from build123d import *

# Parameters (mm, degrees)
CYLINDER001_R     = 8
CYLINDER001_DEPTH = 20
CYLINDER_R        = 11.2
CYLINDER_DEPTH    = 10


with BuildPart() as cylinder001:
    # Cylinder001 → Cylinder001 (new body)
    with BuildSketch(Plane.XY):
        Circle(CYLINDER001_R)
    extrude(amount=CYLINDER001_DEPTH)


with BuildPart() as cylinder:
    # Cylinder → Cylinder (new body)
    with BuildSketch(Plane.XY):
        Circle(CYLINDER_R)
    extrude(amount=CYLINDER_DEPTH)


with BuildPart() as cut001:
    # Cone → Cone (revolve)
    with BuildSketch(Plane.XZ):
        Polygon((0, 0), (20, 0), (12, 20), (0, 20), align=None)
    revolve(axis=Axis((0, 0, 0), (0, 0, 1)))

    # Cut: cut Cylinder
    add(cylinder.part, mode=Mode.SUBTRACT)

    # Cut001: cut Cylinder001
    add(cylinder001.part, mode=Mode.SUBTRACT)


solid = cut001.part
Source: CAD feature listing. Evaluate the final solid. Frame: model axes, mm. A direction names the side the tool comes from. Coordinates: 2 decimals unless noted, no trailing zeros. Loops run counter-clockwise (first coordinate to the right, second up) from the corner with the lowest first, then second, coordinate; pieces in that order, holes last. Notation, with made-up numbers: (60.25, 1.5) - (85.25, 1.5) arc R32 cw to (85.25, 29.5) - close; hole circle Ø5 at (-32, 43). An arc over 180 degrees is marked (long way). One line per item, written item: value. Start each with the question number.
1. Section A-A (y = 0). Return the cut outline in (x, z).
2. Set-up query: faces 4 (the cylindrical face through (-1.73, -7.81, 14.93)), 5 (the cylindrical face through (-11.19, 0.49, 4.93)). Return all of +Z, -Z, +X, -X, +Y, -Y with unobstructed straight access to the full face (end or side cutting, diameter ignored); none if empty.
3. Contact query for flat-ended pins moving along their axis: P1, Ø6, axis at y = -9.5, z = 16, coming from the +X side; P2, Ø6, axis at x = 10, y = -14, coming from the +Z side; P3, Ø6, axis at x = 1, z = 4, coming from the -Y side; P4, Ø13.5, axis at x = 0, y = 0, coming from the -Z side. Output: stop coordinate, or through.
4. Mould query, pull axis X, two halves, no side actions, for faces 1 (the flat face through (-8, 3, 10)), 2 (the conical face through (-3.07, -13.83, 14.58)), 3 (the flat face through (2, -8, 20)). Classes: pulls with the +X half, pulls with the -X half, needs draft (parallel to the pull), parting line crosses it, or undercut.
5. Section C-C (z = 7.5). Return the cut outline in (x, y), and give its area (3 significant figures).
6. Ray query, L1, parallel to Z at x = -7, y = 8; L2, parallel to Y at x = -9.5, z = 2.75; L3, parallel to X at y = 9, z = 12.5. Return the intervals inside material, ascending.
Verdict:
1. outline: (-20, 0) - (-11.2, 0) - (-11.2, 10) - (-8, 10) - (-8, 20) - (-12, 20) - close; (8, 10) - (11.2, 10) - (11.2, 0) - (20, 0) - (12, 20) - (8, 20) - close
2. face 4: +Z, -Z
2. face 5: -Z
3. P1: stops at x = 12.44
3. P2: stops at z = 14.49
3. P3: stops at y = -19.58
3. P4: passes through
4. face 1: undercut
4. face 2: parting line crosses it
4. face 3: needs draft
5. outline: circle Ø34 at (0, 0); hole circle Ø22.4 at (0, 0)
5. area: 514 mm2
6. L1: z = 10 to 20
6. L2: y = -16.34 to -5.93, 5.93 to 16.34
6. L3: x = -12 to 12
